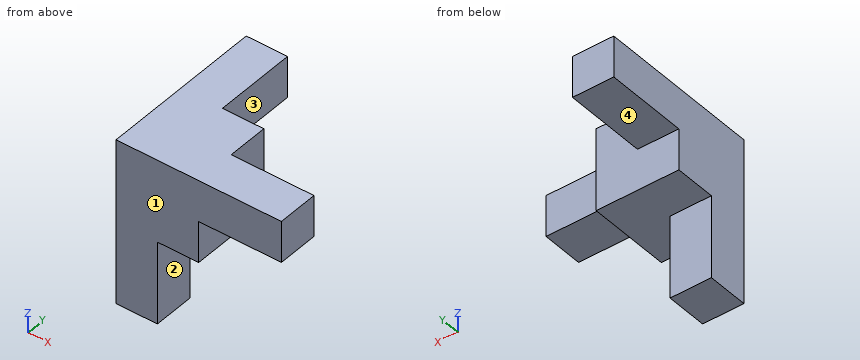
from build123d import *

# Parameters (mm, degrees)
BOSS_EXTRUDE1_DEPTH = 10
SKETCH2_W           = 10
SKETCH2_H           = 10
BOSS_EXTRUDE2_DEPTH = 30
SKETCH3_W           = 20
SKETCH3_H           = 20
BOSS_EXTRUDE3_DEPTH = 20


with BuildPart() as part:
    # Sketch1 → Boss-Extrude1 (new body)
    with BuildSketch(Plane.XY):
        Polygon((0, 0), (10, 0), (40, 0), (40, 10), (10, 10), (10, 40), (0, 40), align=None)
    extrude(amount=BOSS_EXTRUDE1_DEPTH)

    # Sketch2 → Boss-Extrude2 (add)
    with BuildSketch(Plane(origin=(0, 0, 0), x_dir=(-1, 0, 0), z_dir=(0, 0, -1))):
        with Locations((-5, 5)):
            Rectangle(SKETCH2_W, SKETCH2_H)
    extrude(amount=BOSS_EXTRUDE2_DEPTH)

    # Sketch3 → Boss-Extrude3 (add)
    with BuildSketch(Plane.XY.offset(10)):
        with Locations((10, 10)):
            Rectangle(SKETCH3_W, SKETCH3_H)
    extrude(amount=-BOSS_EXTRUDE3_DEPTH)


solid = part.part
Could you check a few things on this model? Use its own coordinates, in mm. Face numbers are marked on the shaded views. A direction names the side the tool comes from. Coordinates: 2 decimals unless noted, no trailing zeros. Order: outer loops, then holes, each group sorted by start corner. A loop starts at its lowest first (then second) coordinate and runs counter-clockwise, first axis right, second up.
Q1. Which directions (+Z, -Z, +X, -X, +Y, -Y) give clear straight access to the entire face, cutting with the end or side of a thin tool? Please do the marked faces 1, 2, 3 and 4.
Q2. Will these pins go through, and if not, where does the flat tip stop? pin 1 (6 mm diameter, centred on x = 26.5, y = 5, fed in from -Z); pin 2 (3 mm diameter, centred on x = 7.5, z = -18.5, fed in from +Y); pin 3 (12 mm diameter, centred on x = 32.5, y = 16.5, fed in from -Z); pin 4 (5 mm diameter, centred on y = 5, z = -18.5, fed in from +X).
Q3. Suppose I cut it at A-A on x = 7.5. Please give me the cut outline in (y, z).
Q4. Suppose I cut it at C-C on y = 21.5. Please give me the cut outline in (x, z).
Q5. Suppose I cut it at B-B on z = 2. Please give me the cut outline in (x, y), and give its area (3 significant figures).
Q6. Suppose I cut it at D-D on z = -7.5. Please give me the cut outline in (x, y), and give its area (3 significant figures).
Q7. Please list where these lines run through material, in increasing order: L1, parallel to X at y = 27.5, z = 8.5; L2, parallel to X at y = 15.5, z = -9.
Answer:
1. face 1: +Z, -Z, +X, -X, -Y
1. face 2: -Z, +X, +Y, -Y
1. face 3: +Z, -Z, +X, +Y
1. face 4: -Z, +X, -X, +Y
2. pin 1: stops at z = 0
2. pin 2: stops at y = 10
2. pin 3: passes through
2. pin 4: stops at x = 10
3. outline: (0, -30) - (10, -30) - (10, -10) - (20, -10) - (20, 0) - (40, 0) - (40, 10) - (0, 10) - close
4. outline: (0, 0) - (10, 0) - (10, 10) - (0, 10) - close
5. outline: (0, 0) - (40, 0) - (40, 10) - (20, 10) - (20, 20) - (10, 20) - (10, 40) - (0, 40) - close
5. area: 800 mm2
6. outline: (0, 0) - (20, 0) - (20, 20) - (0, 20) - close
6. area: 400 mm2
7. L1: x = 0 to 10
7. L2: x = 0 to 20
